from build123d import *

# Parameters (mm, degrees)
SKETCH_2_R               = 70
SKETCH_2_R_2             = 57
EXTRUDE_1_DEPTH          = 12
SKETCH_3_R               = 57
SKETCH_3_R_2             = 40
EXTRUDE_2_DEPTH          = 7
EXTRUDE_START            = 8
SKETCH_4_R               = 95
SKETCH_4_R_2             = 40
EXTRUDE_3_DEPTH          = 8
EXTRUDE_4_DEPTH          = 5
PATTERN_CIRCULAR_2_COUNT = 6
FILLET_1_R               = 3
SKETCH_6_R               = 40
SKETCH_6_R_2             = 32.5
EXTRUDE_5_DEPTH          = 22
SKETCH_7_R               = 45
SKETCH_7_R_2             = 30
EXTRUDE_6_DEPTH          = 12


with BuildPart() as part:
    # Sketch 1 → Revolve 2 (revolve)
    with BuildSketch(Plane(origin=(0, 0, 0), x_dir=(0, 0, -1), z_dir=(1, 0, 0)), mode=Mode.PRIVATE) as revolve_2_sk:
        Polygon((-70, 100), (0, 100), (0, 58), (-9.5, 58), (-9.5, 70), (-70, 70), align=None)
    revolve(revolve_2_sk.sketch.rotate(Axis((0, 0, 1000), (0, 0, -1)), 90), axis=Axis((0, 0, 1000), (0, 0, -1)))



with BuildPart() as body_2:
    # Sketch 2 → Extrude 1 (new body)
    with BuildSketch(Plane.XY.offset(70)):
        Circle(SKETCH_2_R)
        Circle(SKETCH_2_R_2, mode=Mode.SUBTRACT)
    extrude(amount=-EXTRUDE_1_DEPTH)


with BuildPart() as part_1:
    add(part.part)

    add(body_2.part)  # Extrude 2 merges body 2
    # Sketch 3 → Extrude 2 (add)
    with BuildSketch(Plane.XY.offset(70)):
        Circle(SKETCH_3_R)
        Circle(SKETCH_3_R_2, mode=Mode.SUBTRACT)
    extrude(amount=-EXTRUDE_2_DEPTH)

    # Sketch 4 → Extrude 3 (add)
    with BuildSketch(Plane.XY.offset(70).offset(EXTRUDE_START)):
        with Locations(Location((0, 0, 0), (0, 0, 180))):
            Circle(SKETCH_4_R)
        Circle(SKETCH_4_R_2, mode=Mode.SUBTRACT)
    extrude(amount=-EXTRUDE_3_DEPTH)

    # Sketch 5 → Extrude 4 (add)
    with BuildSketch(Plane.XY.offset(78)):
        Polygon((3.464101615, 77), (6.92820323, 83), (3.464101615, 89), (-3.464101615, 89), (-6.92820323, 83), (-3.464101615, 77), align=None)
    extrude_4 = extrude(amount=EXTRUDE_4_DEPTH)

    # Pattern Circular 2: Extrude 4 ×6 about axis
    pattern_circular_2_axis = Axis((0, 0, 0), (0, 0, 1))
    for i in range(1, PATTERN_CIRCULAR_2_COUNT):
        add(extrude_4.rotate(pattern_circular_2_axis, i * 360 / PATTERN_CIRCULAR_2_COUNT))

    # Fillet 1
    fillet_1_edges = [part_1.edges().sort_by_distance(p)[0] for p in [
        (-100, 0, 70),
    ]]
    fillet(fillet_1_edges, radius=FILLET_1_R)

    # Mirror 8: part across plane


with BuildPart() as part_2:
    add(part_1.part)
    add(part_1.part.mirror(Plane(origin=(0, 100, 0), x_dir=(1, 0, 0), z_dir=(0, 0, 1))))

    # Sketch 6 → Extrude 5 (add)
    with BuildSketch(Plane.XY.offset(80)):
        Circle(SKETCH_6_R)
        Circle(SKETCH_6_R_2, mode=Mode.SUBTRACT)
    extrude(amount=-EXTRUDE_5_DEPTH)

    # Sketch 7 → Extrude 6 (add)
    with BuildSketch(Plane.XY.offset(80)):
        Circle(SKETCH_7_R)
        Circle(SKETCH_7_R_2, mode=Mode.SUBTRACT)
    extrude(amount=EXTRUDE_6_DEPTH)


solid = part_2.part
CAD build for the part. Positions are in the model's coordinates, mm. A direction names the side the tool comes from. Coordinates: 2 decimals unless noted, no trailing zeros. Order: outer loops, then holes, each group sorted by start corner. A loop starts at its lowest first (then second) coordinate and runs counter-clockwise, first axis right, second up. Notation, with made-up numbers: (47, 89.25) -> (70, 89.25) arc R28 ccw to (70, 111.25) -> close; hole circle Ø10 at (19, 53.25). An arc over 180 degrees is marked (long way). Answer in a Markdown table with one row per item.
1) Band-saw the part on A-A (z = 37). List the corners of the cut face in (x, y).
Check values:
| item | result |
|---|---|
| outline | circle Ø200 at (0, 0); hole circle Ø140 at (0, 0) |
2) Flat gauge pins, fed straight in: P1, Ø6, axis at x = -2.5, y = 81, coming from the +Z side; P2, Ø1.5, axis at x = 73, z = -81.5, coming from the +Y side; P3, Ø4, axis at x = 72, z = -79.5, coming from the -Y side. Where does each tip first touch, or does it go through?
Check values:
| item | result |
|---|---|
| P1 | z = 83 |
| P2 | y = 47.5 |
| P3 | y = -63.48 |
3) Drill centre lines: line 1 (Y direction, x = 0, z = 61); line 2 (Z direction, x = 63.5, y = -14.5); line 3 (Y direction, x = 0, z = 87.75). Where is each one in solid material? Low to high.
Check values:
| item | result |
|---|---|
| line 1 | -100 to -57, -40 to -32.5, 32.5 to 40, 57 to 100 |
| line 2 | -78 to -58, -9.5 to 9.5, 58 to 78 |
| line 3 | -45 to -30, 30 to 45 |
4) Band-saw the part on B-B (y = 64.5). Give the number of separate pieces and of enclosed holes in the cut face, and give its area (3 significant figures).
Check values:
| item | result |
|---|---|
| separate pieces | 1 |
| enclosed holes | 2 |
| area | 18,300 mm2 |
5) Mould opens along Y. For faces 6 (the face through (77.1, 44.46, -80.46)), 7 (the face through (-5.172, -79.958, 80.465)), 8 (the face through (77.052, -44.542, -80.465)) say: pulls with the +Y half, pulls with the -Y half, needs draft (parallel to the pull), parting line crosses it, or undercut.
Check values:
| item | result |
|---|---|
| face 6 | pulls with the +Y half |
| face 7 | undercut |
| face 8 | pulls with the -Y half |
6) Which spindle directions (+Z, -Z, +X, -X, +Y, -Y) get a long thin tool onto all of the face, cutting with end or side? Do faces 1 (the face through (-72, 47.5, 80)), 2 (the face through (5.172, 79.958, 80.465)), 3 (the face through (71, -64, -70)), 4 (the face through (-5.172, 86.042, -80.465)), 5 (the face through (20.59, 92.74, 74.06)). Say none if no direction does.
Check values:
| item | result |
|---|---|
| face 1 | +Z, +X, -X, +Y |
| face 2 | +Z, +X |
| face 3 | -Z |
| face 4 | -Z, -X, +Y |
| face 5 | +Z |
